For this review, take the finished solid that the model builds, in its own axes (mm). A direction names the side the tool comes from. Coordinates: 2 decimals unless noted, no trailing zeros. Loops run counter-clockwise (first coordinate to the right, second up) from the corner with the lowest first, then second, coordinate; pieces in that order, holes last. Notation, with made-up numbers: M -9,-30.5 L 22,-30.5 A20 cw 22,-5.5 Z; hole C 12,79 d2. An arc over 180 degrees is marked long. Use one line per item in the form item = value.
Autodesk Inventor part; units mm, degrees
ref_plane "YZ Plane" through (0, 0, 0) normal (1, 0, 0) x (0, 1, 0)
ref_plane "XZ Plane" through (0, 0, 0) normal (0, 1, 0) x (-1, 0, 0)
ref_plane "XY Plane" through (0, 0, 0) normal (0, 0, 1) x (1, 0, 0)
sketch "Sketch1" plane through (0, 0, 0) normal (0, 0, 1) x (1, 0, 0)
  line L0 (0, 0) -> (50.8, 0)
  line L1 (50.8, 0) -> (50.8, 25.4)
  line L2 (0, 25.4) -> (0, 0)
  line L3 (3.175, 3.175) -> (47.625, 3.175)
  line L4 (47.625, 3.175) -> (47.625, 25.4)
  line L5 (3.175, 25.4) -> (3.175, 3.175)
  line L6 (0, 25.4) -> (3.175, 25.4)
  line L7 (47.625, 25.4) -> (50.8, 25.4)
  dimension "d0" = 50.8
  dimension "d1" = 25.4
  dimension "d2" = 3.175
  dimension "d3" = 3.175
  dimension "d5" = 3.175
extrude "Extrusion1" add sketch "Sketch1" along normal blind 431.8
sketch "Sketch2" plane through (50.8, 0, 0) normal (1, 0, 0) x (0, 0, -1)
  line L0 (0, 0) -> (0, 25.4)
  line L1 (0, 25.4) -> (-431.8, 25.4)
  circle A0 centre (-12.7, 12.7) radius 6.35
  dimension "d8" = 12.7
  dimension "d9" = 12.7
  dimension "d10" = 12.7
extrude "Extrusion2" cut sketch "Sketch2" against normal blind 431.8
equation "\"d2\" = d5"
equation "\"d5\" = d4"
equation "\"d4\" = d3"
properties part number "shooter U frame"
1. Consider section C-C on z = 333. Write out the cut boundary in (x, y) (3 decimals).
Computed values:
outline = M 0,0 L 50.8,0 L 50.8,25.4 L 47.625,25.4 L 47.625,3.175 L 3.175,3.175 L 3.175,25.4 L 0,25.4 Z
2. Draft analysis for pull direction X (two halves, no side actions). For faces 1 (the face through (1.61, 18.054, 9.286)), 2 (the face through (0, 13, 213)), 3 (the face through (25, 3.175, 213)), state which applies: +X half, -X half, draft (parallel to the pull), parting line (faces both ways), or undercut.
Computed values:
face_1 = draft
face_2 = -X half
face_3 = undercut
3. Wall thickness on line 1 along X through (y, z) = (4.5, 234) (3 decimals); line 2 along Y through (x, z) = (48.65, 12.7); line 3 along Y through (x, z) = (40, 274) (3 decimals): over which ranges is each line inside the solid? List them lowest first. Write a range as from..to.
Computed values:
line_1 = 0..3.175, 47.625..50.8
line_2 = 0..6.35, 19.05..25.4
line_3 = 0..3.175
4. Consider section A-A on z = 12.7. Write out the cut boundary in (x, y) (3 decimals), plus the area to 3 significant figures.
Computed values:
outline = M 0,0 L 50.8,0 L 50.8,6.35 L 47.625,6.35 L 47.625,3.175 L 3.175,3.175 L 3.175,6.35 L 0,6.35 Z; M 0,19.05 L 3.175,19.05 L 3.175,25.4 L 0,25.4 Z; M 47.625,19.05 L 50.8,19.05 L 50.8,25.4 L 47.625,25.4 Z
area = 222 mm2
5. Tool access review of faces 4 (the face through (47.625, 14, 213)), 5 (the face through (27, 2, 431.8)): name each direction out of +Z, -Z, +X, -X, +Y, -Y from which nothing blocks a thin tool from reaching the whole face with its end or side.
Computed values:
face_4 = +Z, -Z, +Y
face_5 = +Z, +X, -X, +Y, -Y
6. Consider section B-B on y = 12.7. Write out the cut boundary in (x, z) (3 decimals), plus the area to 3 significant figures.
Computed values:
outline = M 0,0 L 3.175,0 L 3.175,6.35 L 0,6.35 Z; M 0,19.05 L 3.175,19.05 L 3.175,431.8 L 0,431.8 Z; M 47.625,0 L 50.8,0 L 50.8,6.35 L 47.625,6.35 Z; M 47.625,19.05 L 50.8,19.05 L 50.8,431.8 L 47.625,431.8 Z
area = 2,660 mm2
7. Consider section D-D on x = 27.5. Write out the cut boundary in (y, z) (3 decimals).
Computed values:
outline = M 0,0 L 3.175,0 L 3.175,431.8 L 0,431.8 Z
8. For pin 1 Ø22 at (x, z) = (23, 293) entering from +Y (3 decimals), flat-tipped, find the tip position at first contact; note if it passes through.
Computed values:
pin_1 = 3.175
